```python
from build123d import *

# Parameters (mm, degrees)
SKETCH1_R           = 30
BOSS_EXTRUDE1_DEPTH = 1
SKETCH2_R           = 24.335851471
BOSS_EXTRUDE2_DEPTH = 29
SKETCH3_R           = 5.664148529
BOSS_EXTRUDE3_DEPTH = 29
SKETCH4_R           = 30
BOSS_EXTRUDE4_DEPTH = 1
SKETCH5_R           = 4.681501742
CUT_EXTRUDE1_DEPTH  = 1
SKETCH6_R           = 4.678679428
CUT_EXTRUDE2_DEPTH  = 1


with BuildPart() as part:
    # Sketch1 → Boss-Extrude1 (new body)
    with BuildSketch(Plane(origin=(0, 0, 0), x_dir=(0, 0, -1), z_dir=(1, 0, 0))):
        Circle(SKETCH1_R)
    extrude(amount=BOSS_EXTRUDE1_DEPTH)

    # Sketch2 → Boss-Extrude2 (add)
    with BuildSketch(Plane(origin=(1, 0, 0), x_dir=(0, 0, -1), z_dir=(1, 0, 0))):
        Circle(SKETCH2_R)
    extrude(amount=BOSS_EXTRUDE2_DEPTH)

    # Sketch3 → Boss-Extrude3 (add)
    with BuildSketch(Plane(origin=(30, 0, 0), x_dir=(0, 0, -1), z_dir=(1, 0, 0))):
        with Locations((0, 24.335851471)):
            Circle(SKETCH3_R)
        with Locations((12.167925735, 21.075465597)):
            Circle(SKETCH3_R)
        with Locations((21.075465597, 12.167925735)):
            Circle(SKETCH3_R)
        with Locations((24.335851471, 0)):
            Circle(SKETCH3_R)
        with Locations((21.075465597, -12.167925735)):
            Circle(SKETCH3_R)
        with Locations((12.167925735, -21.075465597)):
            Circle(SKETCH3_R)
        with Locations((0, -24.335851471)):
            Circle(SKETCH3_R)
        with Locations((-12.167925735, -21.075465597)):
            Circle(SKETCH3_R)
        with Locations((-21.075465597, -12.167925735)):
            Circle(SKETCH3_R)
        with Locations((-24.335851471, 0)):
            Circle(SKETCH3_R)
        with Locations((-21.075465597, 12.167925735)):
            Circle(SKETCH3_R)
        with Locations((-12.167925735, 21.075465597)):
            Circle(SKETCH3_R)
    extrude(amount=-BOSS_EXTRUDE3_DEPTH)

    # Sketch4 → Boss-Extrude4 (add)
    with BuildSketch(Plane(origin=(30, 0, 0), x_dir=(0, 0, -1), z_dir=(1, 0, 0))):
        Circle(SKETCH4_R)
    extrude(amount=BOSS_EXTRUDE4_DEPTH)

    # Sketch5 → Cut-Extrude1 (cut)
    with BuildSketch(Plane.ZY):
        Circle(SKETCH5_R)
    extrude(amount=-CUT_EXTRUDE1_DEPTH, mode=Mode.SUBTRACT)

    # Sketch6 → Cut-Extrude2 (cut)
    with BuildSketch(Plane(origin=(31, 0, 0), x_dir=(0, 0, -1), z_dir=(1, 0, 0))):
        Circle(SKETCH6_R)
    extrude(amount=-CUT_EXTRUDE2_DEPTH, mode=Mode.SUBTRACT)


solid = part.part
```
Part model, mm, in its own coordinate system. A direction names the side the tool comes from. Give positions to 0.01 mm unless a question says otherwise; leave off trailing zeros. Order: outer loops, then holes, each group sorted by start corner. A loop starts at its lowest first (then second) coordinate and runs counter-clockwise, first axis right, second up. Notation, with made-up numbers: M 66,-40 L 96,-40 A25 cw 96,-17 Z; hole C -22.5,21 d6. An arc over 180 degrees is marked long. Use a Markdown table: item, result. Add a question column.
(1) Saw through at C-C, the plane z = -22.5. Give the cut face in (x, y), and give its area (3 significant figures).
(2) 3-axis set-ups, long thin cutter, end or side, ignore diameter. For faces 3 (the face through (15.7, -26.05, -14.88)), 4 (the face through (30, 0, 0)), 5 (the face through (1, 0, 0)): which of +Z, -Z, +X, -X, +Y, -Y reach the whole face in a straight line?
(3) Saw through at A-A, the plane x = 14. Give the cut face in (y, z).
(4) Drop flat-ended pins along their axis: P1, Ø1.5, axis at x = 4.5, y = 7.5, coming from the +Z side; P2, Ø7.5, axis at y = 0, z = 0, coming from the -X side; P3, Ø1.5, axis at x = 14, z = 4, coming from the -Y side. Give the stop position or say it passes through.
(5) Saw through at B-B, the plane y = 19. Give the cut face in (x, z), and give its area (3 significant figures).
(6) Mould opens along Y. For faces 1 (the face through (30, 27, 8)), 2 (the face through (1, 8, 27)) say: +Y half, -Y half, draft (parallel to the pull), parting line (faces both ways), or undercut.
(7) Probe line 1 along Y through (x, z) = (3, -25.5); line 2 along X through (y, z) = (5.5, -28). List the from-to ranges inside material, lowest first. Write a range as [from, to].
Answer key:
| question | item | result |
|---|---|---|
| 1 | outline | M 0,-19.84 L 1,-19.84 L 1,-17.65 L 30,-17.65 L 30,-19.84 L 31,-19.84 L 31,19.84 L 30,19.84 L 30,17.65 L 1,17.65 L 1,19.84 L 0,19.84 Z |
| 1 | area | 1,100 mm^2 |
| 2 | face 3 | none |
| 2 | face 4 | +X |
| 2 | face 5 | -X |
| 3 | outline | M -23.68,-5.63 A24.34 ccw -23.32,-6.97 A5.66 ccw long -17.69,-16.71 A24.34 ccw -16.71,-17.69 A5.66 ccw long -6.97,-23.32 A24.34 ccw -5.63,-23.68 A5.66 ccw long 5.63,-23.68 A24.34 ccw 6.97,-23.32 A5.66 ccw long 16.71,-17.69 A24.34 ccw 17.69,-16.71 A5.66 ccw long 23.32,-6.97 A24.34 ccw 23.68,-5.63 A5.66 ccw long 23.68,5.63 A24.34 ccw 23.32,6.97 A5.66 ccw long 17.69,16.71 A24.34 ccw 16.71,17.69 A5.66 ccw long 6.97,23.32 A24.34 ccw 5.63,23.68 A5.66 ccw long -5.63,23.68 A24.34 ccw -6.97,23.32 A5.66 ccw long -16.71,17.69 A24.34 ccw -17.69,16.71 A5.66 ccw long -23.32,6.97 A24.34 ccw -23.68,5.63 A5.66 ccw long Z |
| 4 | P1 | z = 25.17 |
| 4 | P2 | x = 1 |
| 4 | P3 | y = -28.97 |
| 5 | outline | M 0,-23.22 L 1,-23.22 L 1,-17.44 L 30,-17.44 L 30,-23.22 L 31,-23.22 L 31,23.22 L 30,23.22 L 30,17.44 L 1,17.44 L 1,23.22 L 0,23.22 Z |
| 5 | area | 1,100 mm^2 |
| 6 | face 1 | draft |
| 6 | face 2 | undercut |
| 7 | line 1 | [-15.7, -8.63], [-5.54, 5.54], [8.63, 15.7] |
| 7 | line 2 | [0, 1], [30, 31] |
